from build123d import *

# Parameters (mm, degrees)
F0_W     = 50.8
F0_H     = 50.8
F1_DEPTH = 50.8
F2_T     = -12.7
F3_R     = 6.35
F4_DEPTH = 25.4
F5_R     = 6.34999


# Not quite as in the source:
# - a fillet or chamfer is up to 0.001 mm smaller than in the source, because OpenCascade refuses the exact size


with BuildPart() as f1:
    # F0 (on Right) → F1 (new body)
    with BuildSketch(Plane.YZ):
        Rectangle(F0_W, F0_H)
    extrude(amount=F1_DEPTH)

    # F2
    f2_openings = [f1.faces().sort_by_distance(p)[0] for p in [
        (25.4, 0, 25.4),
        (25.4, 0, -25.4),
    ]]
    offset(amount=F2_T, openings=f2_openings)

    # F3 (on face) → F4 (join)
    with BuildSketch(Plane(origin=(0, 0, 0), x_dir=(0, -1, 0), z_dir=(-1, 0, 0))):
        Circle(F3_R)
    extrude(amount=F4_DEPTH)

    # F5 (radius 6.35 in the source; OpenCascade refuses exactly that, so slightly less here)
    f5_edges = [f1.edges().sort_by_distance(p)[0] for p in [
        (50.8, -25.4, 0),
        (0, -25.4, 0),
        (50.8, 25.4, 0),
        (0, 25.4, 0),
        (12.7, -12.7, 0),
        (38.1, 12.7, 0),
        (12.7, 12.7, 0),
        (38.1, -12.7, 0),
        (25.4, 25.4, 25.4),
        (50.8, 0, 25.4),
        (25.4, -25.4, 25.4),
        (0, 0, 25.4),
        (25.4, 12.7, 25.4),
        (12.7, 0, 25.4),
        (25.4, -12.7, 25.4),
        (38.1, 0, 25.4),
        (25.4, -25.4, -25.4),
        (50.8, 0, -25.4),
        (25.4, 25.4, -25.4),
        (0, 0, -25.4),
        (25.4, -12.7, -25.4),
        (12.7, 0, -25.4),
        (25.4, 12.7, -25.4),
        (38.1, 0, -25.4),
    ]]
    fillet(f5_edges, radius=F5_R)


solid = f1.part
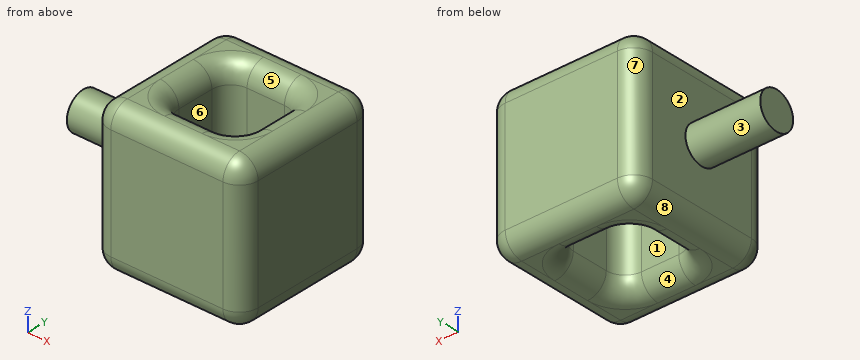
Work out the finished part from the listing and answer in its coordinate system (mm). Face numbers are marked on the shaded views. A direction names the side the tool comes from. Give positions to 0.01 mm unless a question says otherwise; leave off trailing zeros. Order: outer loops, then holes, each group sorted by start corner. A loop starts at its lowest first (then second) coordinate and runs counter-clockwise, first axis right, second up. Notation, with made-up numbers: M 16,35.5 L 28,35.5 A8 ccw 28,41.5 Z; hole C -3,45.5 d8. An arc over 180 degrees is marked long. Return JSON: item names as keys, results as strings.
Q1. Find section C-C, the plane z = 0. Write down the section's boundary in (x, y).
Answer below:
{"outline": "M -25.4,-6.35 L 0,-6.35 L 0,-19.05 A6.35 ccw 6.35,-25.4 L 44.45,-25.4 A6.35 ccw 50.8,-19.05 L 50.8,19.05 A6.35 ccw 44.45,25.4 L 6.35,25.4 A6.35 ccw 0,19.05 L 0,6.35 L -25.4,6.35 Z; hole M 12.7,-6.35 A6.35 ccw 19.05,-12.7 L 31.75,-12.7 A6.35 ccw 38.1,-6.35 L 38.1,6.35 A6.35 ccw 31.75,12.7 L 19.05,12.7 A6.35 ccw 12.7,6.35 Z"}
Q2. Each of these flat-tipped pins is pushed along its axis until it touches: pin 1 (10 mm diameter, centred on x = 1.5, z = -13.5, fed in from +Y); pin 2 (2 mm diameter, centred on x = -3.5, z = 2.5, fed in from -Y); pin 3 (8 mm diameter, centred on y = 17.5, z = 7.5, fed in from -X); pin 4 (12 mm diameter, centred on x = -4, z = -15.5, fed in from -Y). Where does it stop, or does it pass through?
Answer below:
{"pin 1": "stops at y = 25.4", "pin 2": "stops at y = -6.17", "pin 3": "stops at x = 0", "pin 4": "stops at y = -23.68"}
Q3. Find the intervals of material crossed by line 1 along Y through (x, z) = (19, 6.5); line 2 along X through (y, z) = (2.5, -5.5); line 3 along X through (y, z) = (-2, -12.5), in increasing order. Write a range as [from, to].
Answer below:
{"line 1": "y = [-25.4, -12.7], [12.7, 25.4]", "line 2": "x = [-25.4, 12.7], [38.1, 50.8]", "line 3": "x = [0, 12.7], [38.1, 50.8]"}
Q4. Which of the six approach directions +Z, -Z, +X, -X, +Y, -Y give full straight-line access (tool end or side, diameter ignored) to the marked faces 4, 5, 6, 7 and 8?
Answer below:
{"face 4": "-Z", "face 5": "+Z", "face 6": "+Z, -Z", "face 7": "+Z, -Z, -X, +Y", "face 8": "-Z, -X, +Y, -Y"}
Q5. The mould has two halves that part along X. Classify the marked faces 1, 2 and 3: pulls with the +X half, pulls with the -X half, needs draft (parallel to the pull), parting line crosses it, or undercut.
Answer below:
{"face 1": "undercut", "face 2": "pulls with the -X half", "face 3": "needs draft"}
